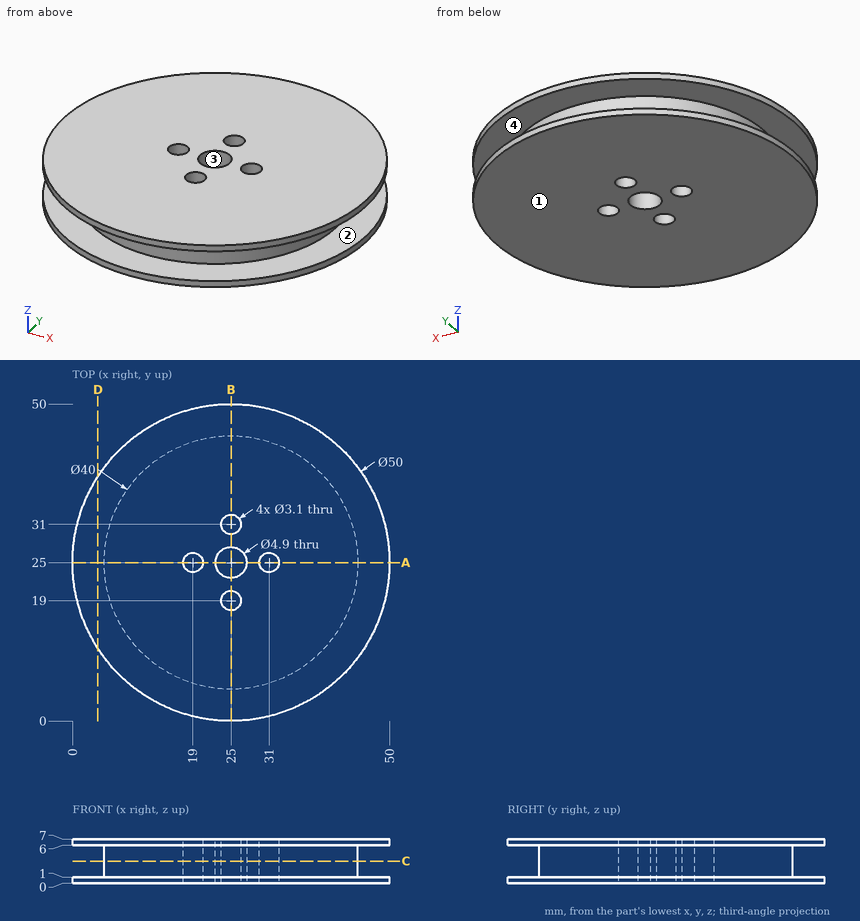
Geometry: see drawing. Coordinates: mm, zero at the bounding-box minimum. A direction names the side the tool comes from. Give positions to 0.01 mm unless a question says otherwise; leave off trailing zeros. Loops run counter-clockwise (first coordinate to the right, second up) from the corner with the lowest first, then second, coordinate; pieces in that order, holes last. Notation, with made-up numbers: (0, -28) - (10, -28) arc R8 ccw to (10, -13) - close; hole circle Ø5 at (28, -0.5). An arc over 180 degrees is marked (long way). One line per question, with ' | ' between items. Start each with the question number.
(1) Contact query for flat-ended pins moving along their axis: pin 1 (4.5 mm diameter, centred on x = 25, y = 25, fed in from +Z); pin 2 (3 mm diameter, centred on x = 35.5, z = 3, fed in from -Y). Output: stop coordinate, or through.
(2) Section query A-A on y = 25. Return loops of the section in (x, z), then the cut area to 3 significant figures.
(3) Reachability of the marked faces 1 and 2 from +Z, -Z, +X, -X, +Y, -Y: full face, straight path, thin tool, end or side. Return the list, or none.
(4) Ray query, line 1 (Y direction, x = 25, z = 4); line 2 (Z direction, x = 44.5, y = 16.5); line 3 (Y direction, x = 26, z = 3.5). Return the intervals inside material, ascending. Write a range as from..to.
(5) Section query C-C on z = 3.5. Return loops of the section in (x, y).
(6) Pull-direction query (Y, two-part tool) for the marked faces 3 and 4; classes: released by +Y, released by -Y, zero draft, split by the parting line, or undercut.
(7) Section query D-D on x = 4. Return loops of the section in (y, z).
The answers:
1) pin 1: through | pin 2: y = 7.14
2) outline: (0, 0) - (17.45, 0) - (17.45, 7) - (0, 7) - (0, 6) - (5, 6) - (5, 1) - (0, 1) - close; (20.55, 0) - (22.55, 0) - (22.55, 7) - (20.55, 7) - close; (27.45, 0) - (29.45, 0) - (29.45, 7) - (27.45, 7) - close; (32.55, 0) - (50, 0) - (50, 1) - (45, 1) - (45, 6) - (50, 6) - (50, 7) - (32.55, 7) - close | area: 222 mm2
3) face 1: -Z, +X, -X, +Y, -Y | face 2: none
4) line 1: 5..17.45, 20.55..22.55, 27.45..29.45, 32.55..45 | line 2: 0..1, 6..7 | line 3: 5.03..17.82, 20.18..22.76, 27.24..29.82, 32.18..44.97
5) outline: circle Ø40 at (25, 25); hole circle Ø3.1 at (19, 25); hole circle Ø4.9 at (25, 25); hole circle Ø3.1 at (25, 19); hole circle Ø3.1 at (25, 31); hole circle Ø3.1 at (31, 25)
6) face 3: undercut | face 4: zero draft
7) outline: (11.44, 0) - (38.56, 0) - (38.56, 1) - (11.44, 1) - close; (11.44, 6) - (38.56, 6) - (38.56, 7) - (11.44, 7) - close
